```python
from build123d import *

# Parameters (mm, degrees)
F0_W      = 50
F0_H      = 27
F1_DEPTH  = 16
F2_W      = 44
F2_H      = 22
F3_DEPTH  = 14
F5_DEPTH  = 12
F6_R      = 1.25
F8_DEPTH  = 14.001
F7_R      = 1.25
F9_DEPTH  = 14.001
F11_DEPTH = 1.8
F13_DEPTH = 2
F14_W     = 4
F14_H     = 0.2
F15_DEPTH = 1
F16_W     = 1.2
F16_H     = 0.5
F16_H_2   = 23
F17_DEPTH = 2
F18_W     = 3.75
F18_H     = 3.75
F19_DEPTH = 4.5
F20_W     = 3.75
F20_H     = 3.75
F21_DEPTH = 4.5
F22_R     = 1.75
F23_DEPTH = 7.501
F24_R     = 1.75
F25_DEPTH = 7.501
F26_R     = 11.25
F27_DEPTH = 29.5


with BuildPart() as f1:
    # F0 (on Top) → F1 (new body)
    with BuildSketch(Plane.XY):
        Rectangle(F0_W, F0_H)
    extrude(amount=F1_DEPTH)

    # F2 (on face) → F3 (cut)
    with BuildSketch(Plane.XY.offset(16)):
        Rectangle(F2_W, F2_H)
    extrude(amount=-F3_DEPTH, mode=Mode.SUBTRACT)

    # F4 (on face) → F5 (join)
    with BuildSketch(Plane.XY.offset(2)):
        with BuildLine():
            ThreePointArc((19.5, -7.25), (21.0909902577, -6.5909902577), (21.75, -5))
            ThreePointArc((21.75, -5), (21.0909902577, -3.4090097423), (19.5, -2.75))
            Line((19.5, -2.75), (19.5, -7.25))
        make_face()
        with BuildLine():
            ThreePointArc((19.5, -2.75), (21.0909902577, -3.4090097423), (21.75, -5))
            ThreePointArc((21.75, -5), (21.0909902577, -6.5909902577), (19.5, -7.25))
            Line((19.5, -7.25), (22, -7.25))
            Line((22, -7.25), (22, -2.75))
            Line((22, -2.75), (19.5, -2.75))
        make_face()
        with BuildLine():
            Line((19.5, -7.25), (19.5, -2.75))
            ThreePointArc((19.5, -2.75), (17.25, -5), (19.5, -7.25))
        make_face()
        with BuildLine():
            Line((-16.75, 8.5), (-12.25, 8.5))
            ThreePointArc((-12.25, 8.5), (-14.5, 10.75), (-16.75, 8.5))
        make_face()
        with BuildLine():
            ThreePointArc((-16.75, 8.5), (-14.5, 6.25), (-12.25, 8.5))
            Line((-12.25, 8.5), (-16.75, 8.5))
        make_face()
        with BuildLine():
            ThreePointArc((-16.75, 8.5), (-14.5, 10.75), (-12.25, 8.5))
            Line((-12.25, 8.5), (-12.25, 11))
            Line((-12.25, 11), (-16.75, 11))
            Line((-16.75, 11), (-16.75, 8.5))
        make_face()
    extrude(amount=F5_DEPTH)

    # F6 (on face) → F8 (cut, through all)
    with BuildSketch(Plane.XY.offset(14)):
        with Locations((-14.5, 8.5)):
            Circle(F6_R)
    extrude(amount=-F8_DEPTH, mode=Mode.SUBTRACT)

    # F7 (on face) → F9 (cut, through all)
    with BuildSketch(Plane.XY.offset(14)):
        with Locations((19.5, -5)):
            Circle(F7_R)
    extrude(amount=-F9_DEPTH, mode=Mode.SUBTRACT)

    # F10 (on face) → F11 (cut)
    with BuildSketch(Plane(origin=(0, 0, 0), x_dir=(1, 0, 0), z_dir=(0, 0, -1))):
        Polygon((-15.6547005384, -10.5), (-13.3452994616, -10.5), (-12.1905989232, -8.5), (-13.3452994616, -6.5), (-15.6547005384, -6.5), (-16.8094010768, -8.5), align=None)
        Polygon((20.6547005384, 7), (18.3452994616, 7), (17.1905989232, 5), (18.3452994616, 3), (20.6547005384, 3), (21.8094010768, 5), align=None)
    extrude(amount=-F11_DEPTH, mode=Mode.SUBTRACT)

    # F12 (on face) → F13 (cut)
    with BuildSketch(Plane.XY.offset(14)):
        with BuildLine():
            Line((22, -2.95), (22, -2.75))
            Line((22, -2.75), (19.5, -2.75))
            ThreePointArc((19.5, -2.75), (19.025658351, -2.8005682552), (18.5726381505, -2.95))
            Line((18.5726381505, -2.95), (22, -2.95))
        make_face()
    extrude(amount=-F13_DEPTH, mode=Mode.SUBTRACT)

    # F14 (on face) → F15 (cut)
    with BuildSketch(Plane.XY.offset(14)):
        with Locations((-14.2456165999, 6.35)):
            Rectangle(F14_W, F14_H)
    extrude(amount=-F15_DEPTH, mode=Mode.SUBTRACT)

    # F16 (on face) → F17 (cut)
    with BuildSketch(Plane.XY.offset(16)):
        Polygon((-22.5, -11.5), (-22.5, -12), (-23.7, -12), (-23.7, -12.7), (23.7, -12.7), (23.7, -12), (22.5, -12), (22.5, -11.5), align=None)
        with Locations((-23.1, -11.75)):
            Rectangle(F16_W, F16_H)
        with Locations((-23.1, 0)):
            Rectangle(F16_W, F16_H_2)
        with Locations((-23.1, 11.75)):
            Rectangle(F16_W, F16_H)
        Polygon((-22.5, 12), (-22.5, 11.5), (22.5, 11.5), (22.5, 12), (23.7, 12), (23.7, 12.7), (-23.7, 12.7), (-23.7, 12), align=None)
        with Locations((23.1, -11.75)):
            Rectangle(F16_W, F16_H)
        with Locations((23.1, 0)):
            Rectangle(F16_W, F16_H_2)
        with Locations((23.1, 11.75)):
            Rectangle(F16_W, F16_H)
    extrude(amount=-F17_DEPTH, mode=Mode.SUBTRACT)

    # F18 (on face) → F19 (join)
    with BuildSketch(Plane(origin=(22, 0, 0), x_dir=(0, -1, 0), z_dir=(-1, 0, 0))):
        with Locations((9.125, 3.875)):
            Rectangle(F18_W, F18_H)
    extrude(amount=F19_DEPTH)

    # F20 (on face) → F21 (join)
    with BuildSketch(Plane.YZ.offset(-22)):
        with Locations((-9.125, 3.875)):
            Rectangle(F20_W, F20_H)
    extrude(amount=F21_DEPTH)

    # F22 (on face) → F23 (cut, through all)
    with BuildSketch(Plane.YZ.offset(-17.5)):
        with Locations((-9.125, 3.875)):
            Circle(F22_R)
    extrude(amount=-F23_DEPTH, mode=Mode.SUBTRACT)

    # F24 (on face) → F25 (cut, through all)
    with BuildSketch(Plane(origin=(17.5, 0, 0), x_dir=(0, -1, 0), z_dir=(-1, 0, 0))):
        with Locations((9.125, 3.875)):
            Circle(F24_R)
    extrude(amount=-F25_DEPTH, mode=Mode.SUBTRACT)

    # F26 (on Right) → F27 (cut, symmetric)
    with BuildSketch(Plane.YZ):
        with Locations((0, -10.25)):
            Circle(F26_R)
    extrude(amount=F27_DEPTH, both=True, mode=Mode.SUBTRACT)


solid = f1.part
```
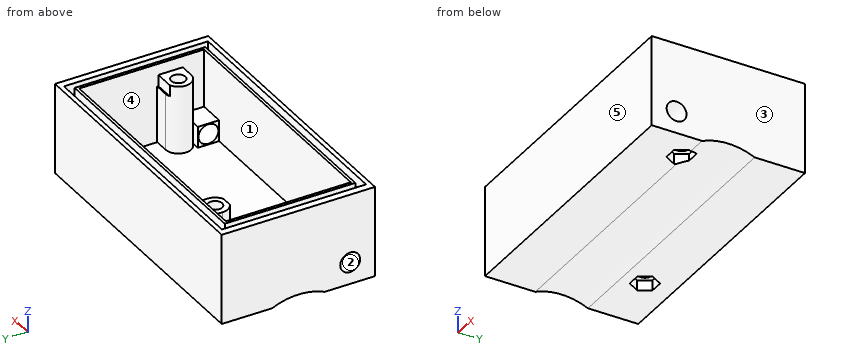
For this review, take the finished solid that the model builds, in its own axes (mm). Face numbers are marked on the shaded views. A direction names the side the tool comes from. Give positions to 0.01 mm unless a question says otherwise; leave off trailing zeros. Order: outer loops, then holes, each group sorted by start corner. A loop starts at its lowest first (then second) coordinate and runs counter-clockwise, first axis right, second up.
1) The part is to be moulded in two halves that separate along Y. For the marked faces 3, 4 and 5, say which applies: released by +Y, released by -Y, zero draft, split by the parting line, or undercut.
2) Insertion check: pin 1 (3 mm diameter, centred on y = -9.125, z = 3.875, fed in from -X). The pin has a flat end and moves straight along its axis. Give the tip position at first contact, or say it passes through.
3) Take a section at B-B (z = 9.25). Give the boundary of the cut face in (x, y).
4) Wall thickness on line 1 (Y direction, x = -14.5, z = 9.5); line 2 (X direction, y = 10.25, z = 7); line 3 (X direction, y = -3.5, z = 15): over which ranges is each line inside the solid? List them lowest first.
5) Take a section at C-C (z = 4.5). Give the boundary of the cut face in (x, y).
6) Take a section at D-D (x = 15.5). Give the boundary of the cut face in (y, z), then the cut area to 3 significant figures.
7) For the marked faces 1 and 2, list the 3-axis set-ups (+Z, -Z, +X, -X, +Y, -Y) from which the entire face can be reached by the end or side of a thin tool; tool diameter is ignored.
Derived:
1. face 3: zero draft
1. face 4: undercut
1. face 5: released by -Y
2. pin 1: passes through
3. outline: (-25, -13.5) - (25, -13.5) - (25, 13.5) - (-25, 13.5) - close; hole (-22, -11) - (22, -11) - (22, -7.25) - (19.5, -7.25) arc R2.25 cw to (19.5, -2.75) - (22, -2.75) - (22, 11) - (-12.25, 11) - (-12.25, 8.5) arc R2.25 cw to (-16.75, 8.5) - (-16.75, 11) - (-22, 11) - close; hole circle Ø2.5 at (-14.5, 8.5); hole circle Ø2.5 at (19.5, -5)
4. line 1: y = -13.5 to -11, 6.25 to 7.25, 9.75 to 13.5
4. line 2: x = -25 to -22, -16.75 to -12.25, 22 to 25
4. line 3: x = -25 to -23.7, -22.5 to -22, 22 to 22.5, 23.7 to 25
5. outline: (-25, -13.5) - (25, -13.5) - (25, -10.76) - (17.5, -10.76) - (17.5, -11) - (-17.5, -11) - (-17.5, -10.76) - (-25, -10.76) - close; (-25, -7.49) - (-17.5, -7.49) - (-17.5, -7.25) - (-22, -7.25) - (-22, 11) - (-16.75, 11) - (-16.75, 8.5) arc R2.25 ccw to (-12.25, 8.5) - (-12.25, 11) - (22, 11) - (22, -2.75) - (19.5, -2.75) arc R2.25 ccw to (19.5, -7.25) - (17.5, -7.25) - (17.5, -7.49) - (25, -7.49) - (25, 13.5) - (-25, 13.5) - close; hole circle Ø2.5 at (-14.5, 8.5); hole circle Ø2.5 at (19.5, -5)
6. outline: (-13.5, 0) - (-4.64, 0) arc R11.25 cw to (4.64, 0) - (13.5, 0) - (13.5, 16) - (12.7, 16) - (12.7, 14) - (11.5, 14) - (11.5, 16) - (11, 16) - (11, 2) - (-11, 2) - (-11, 16) - (-11.5, 16) - (-11.5, 14) - (-12.7, 14) - (-12.7, 16) - (-13.5, 16) - close
6. area: 113 mm2
7. face 1: +Z
7. face 2: +X, -X
